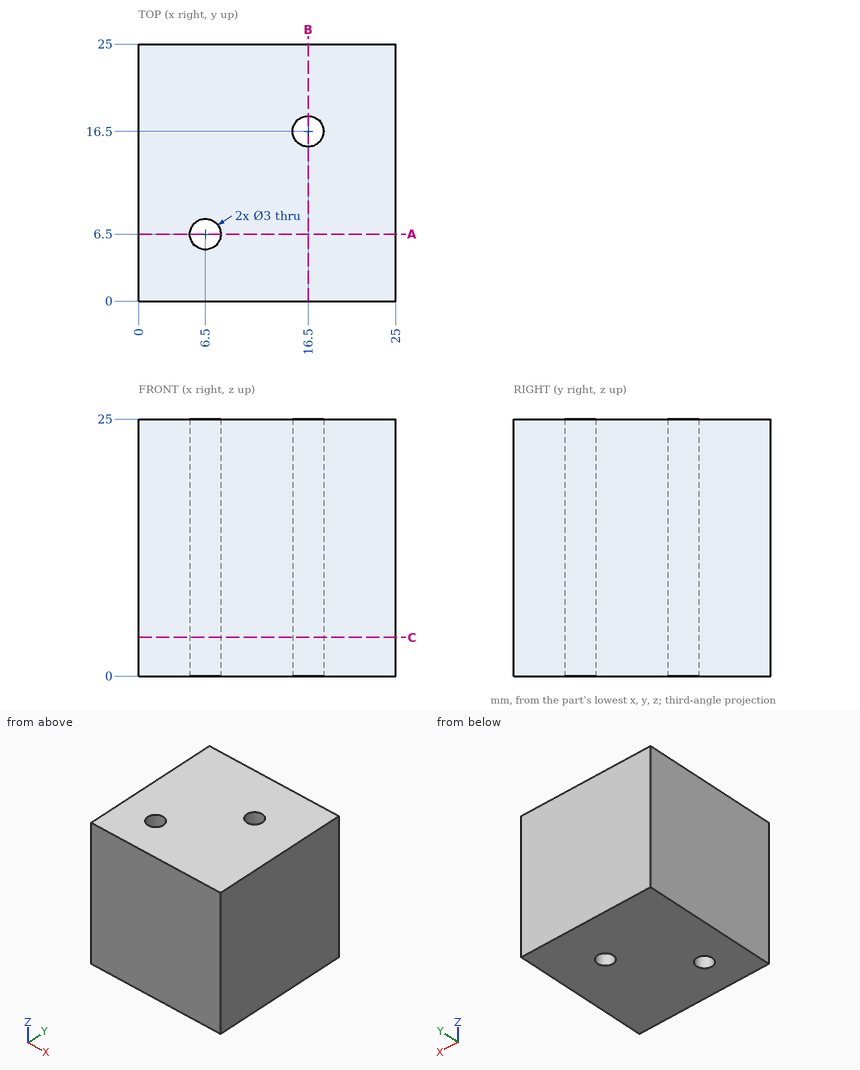
Verification items for this drawing (mm, ordinates from the low corner). Give positions to 0.01 mm unless a question says otherwise; leave off trailing zeros. Loops run counter-clockwise (first coordinate to the right, second up) from the corner with the lowest first, then second, coordinate; pieces in that order, holes last. Notation, with made-up numbers: M -23,12 L 2,12 A7 cw 2,19 Z; hole C 41,-24.75 d2. An arc over 180 degrees is marked long. Write item = value, one per line.
(1) Material ranges on line 1 (Y direction, x = 16.5, z = 12.25); line 2 (Y direction, x = 6.5, z = 18.25); line 3 (X direction, y = 7, z = 17), recorded low to high. Write a range as [from, to].
Answer below:
line_1 = [0, 15], [18, 25]
line_2 = [0, 5], [8, 25]
line_3 = [0, 5.09], [7.91, 25]
(2) Sectioned sample at C-C, the plane z = 3.75. Record the cut outline in (x, y), plus the area to 3 significant figures.
Answer below:
outline = M 0,0 L 25,0 L 25,25 L 0,25 Z; hole C 6.5,6.5 d3; hole C 16.5,16.5 d3
area = 611 mm2
(3) Sectioned sample at A-A, the plane y = 6.5. Record the cut outline in (x, z).
Answer below:
outline = M 0,0 L 5,0 L 5,25 L 0,25 Z; M 8,0 L 25,0 L 25,25 L 8,25 Z
(4) Sectioned sample at B-B, the plane x = 16.5. Record the cut outline in (y, z), plus the area to 3 significant figures.
Answer below:
outline = M 0,0 L 15,0 L 15,25 L 0,25 Z; M 18,0 L 25,0 L 25,25 L 18,25 Z
area = 550 mm2
